Job drawing, mm, ordinate dimensions from the low corner. One solid piece. Coordinates: 2 decimals unless noted, no trailing zeros. Loops run counter-clockwise (first coordinate to the right, second up) from the corner with the lowest first, then second, coordinate; pieces in that order, holes last. Notation, with made-up numbers: (-3, 77) - (16, 77) arc R22 ccw to (16, 86) - close; hole circle Ø4 at (48, -0.75). An arc over 180 degrees is marked (long way). Use a Markdown table: item, result. Add a question column.
1. Band-saw the part on C-C, the plane x = 22.5. Give the cut face in (y, z).
2. Band-saw the part on A-A, the plane y = 125. Give the cut face in (x, z).
3. Band-saw the part on B-B, the plane z = 6.75. Give the cut face in (x, y).
4. Wall check: probe 1 along X at (y, z) = (140, 3.5); probe 2 along Y at (x, z) = (37.5, 6); probe 3 along Y at (x, z) = (20.5, 1.25). Give the ranges that are in metal, low to high. Write a range as [from, to].
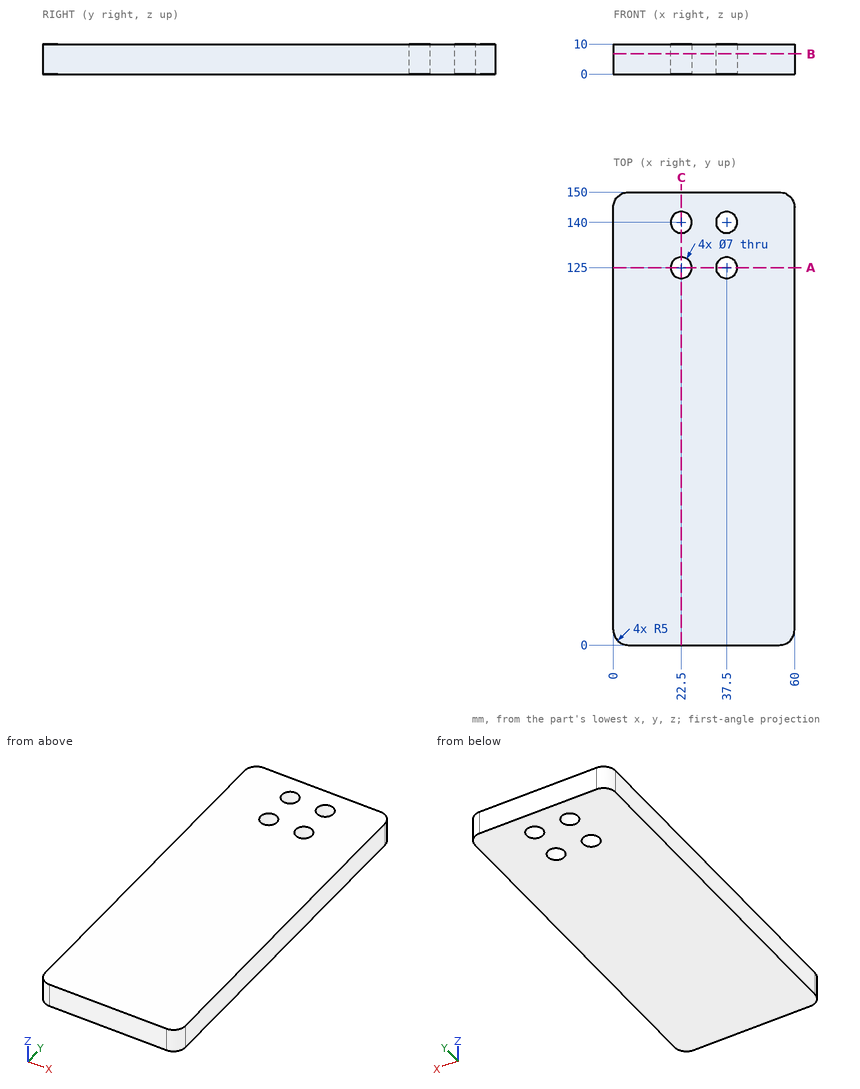
Geometry check:
| question | item | result |
|---|---|---|
| 1 | outline | (0, 0) - (121.5, 0) - (121.5, 10) - (0, 10) - close; (128.5, 0) - (136.5, 0) - (136.5, 10) - (128.5, 10) - close; (143.5, 0) - (150, 0) - (150, 10) - (143.5, 10) - close |
| 2 | outline | (0, 0) - (19, 0) - (19, 10) - (0, 10) - close; (26, 0) - (34, 0) - (34, 10) - (26, 10) - close; (41, 0) - (60, 0) - (60, 10) - (41, 10) - close |
| 3 | outline | (0, 5) arc R5 ccw to (5, 0) - (55, 0) arc R5 ccw to (60, 5) - (60, 145) arc R5 ccw to (55, 150) - (5, 150) arc R5 ccw to (0, 145) - close; hole circle Ø7 at (22.5, 125); hole circle Ø7 at (22.5, 140); hole circle Ø7 at (37.5, 125); hole circle Ø7 at (37.5, 140) |
| 4 | probe 1 | x = [0, 19], [26, 34], [41, 60] |
| 4 | probe 2 | y = [0, 121.5], [128.5, 136.5], [143.5, 150] |
| 4 | probe 3 | y = [0, 122.13], [127.87, 137.13], [142.87, 150] |
